Design review of the part built by this model. Coordinates are the model's own, in mm. A direction names the side the tool comes from. Coordinates: 2 decimals unless noted, no trailing zeros. Write each loop counter-clockwise with the first axis right and the second up, starting at its lowest first coordinate (ties: lowest second). Pieces come first, ordered by that corner, then holes. Notation, with made-up numbers: (-12, -17) -> (17, -17) arc R28 cw to (17, 17) -> close; hole circle Ø4 at (62, 9). An arc over 180 degrees is marked (long way). Write item = value, one per line. Start each with the question number.
```python
from build123d import *

# Parameters (mm, degrees)
SKETCH039_R     = 16.25
PAD017_DEPTH    = 4
POCKET014_DEPTH = 3.4
POCKET015_DEPTH = 0.601
CHAMFER012_SIZE = 0.4


with BuildPart() as part:
    # Sketch039 → Pad017 (new body)
    with BuildSketch(Plane.XY):
        with BuildLine():
            Line((-15.8267662036, 20.9422055079), (-4.8824534392, 29.2132101696))
            ThreePointArc((-4.8824534392, 29.2132101696), (-3.1285346801, 31.3265452468), (-2.5, 34))
            Line((-2.5, 34), (-2.5, 63.75))
            ThreePointArc((2.5, 63.75), (0, 66.25), (-2.5, 63.75))
            Line((2.5, 63.75), (2.5, 34))
            ThreePointArc((2.5, 34), (3.1285346801, 31.3265452468), (4.8824534392, 29.2132101696))
            Line((4.8824534392, 29.2132101696), (15.8267662036, 20.9422055079))
            ThreePointArc((-15.8267662036, 20.9422055079), (0, -26.25), (15.8267662036, 20.9422055079))
        make_face()
        Circle(SKETCH039_R, mode=Mode.SUBTRACT)
    extrude(amount=PAD017_DEPTH)

    # Sketch040 → Pocket014 (cut)
    with BuildSketch(Plane.XY):
        with BuildLine():
            Line((-14.9659183372, 6.3311759039), (-21.4611088655, 10.0811759039))
            ThreePointArc((-19.4611088655, 13.545277519), (-20.5342878135, 11.8554765967), (-21.4611088655, 10.0811759039))
            Line((-19.4611088655, 13.545277519), (-12.9659183372, 9.795277519))
            Line((-12.9659183372, 9.795277519), (-14.9659183372, 6.3311759039))
        make_face()
        with BuildLine():
            Line((-16.2287527148, 0.8307137431), (-23.6148108624, 2.1330750756))
            ThreePointArc((-22.9202181517, 6.0723060876), (-23.3507305362, 4.1173638128), (-23.6148108624, 2.1330750756))
            Line((-22.9202181517, 6.0723060876), (-15.5341600041, 4.7699447551))
            Line((-15.5341600041, 4.7699447551), (-16.2287527148, 0.8307137431))
        make_face()
        with BuildLine():
            Line((-11.8979733346, 11.0680048124), (-16.7188804073, 16.8133381358))
            ThreePointArc((-13.6547026348, 19.3844885746), (-15.2411069266, 18.1636439349), (-16.7188804073, 16.8133381358))
            Line((-13.6547026348, 19.3844885746), (-8.8337955622, 13.6391552512))
            Line((-11.8979733346, 11.0680048124), (-8.8337955622, 13.6391552512))
        make_face()
        with BuildLine():
            Line((-7.3949571526, 14.4698689943), (-9.9601082275, 21.5175636502))
            ThreePointArc((-6.2013377444, 22.8856442235), (-8.1096236096, 22.2810077477), (-9.9601082275, 21.5175636502))
            Line((-6.2013377444, 22.8856442235), (-3.6361866695, 15.8379495676))
            Line((-7.3949571526, 14.4698689943), (-3.6361866695, 15.8379495676))
        make_face()
        with BuildLine():
            Line((-15.5341600041, -4.7699447551), (-22.9202181517, -6.0723060876))
            ThreePointArc((-23.6148108624, -2.1330750756), (-23.3507305362, -4.1173638128), (-22.9202181517, -6.0723060876))
            Line((-23.6148108624, -2.1330750756), (-16.2287527148, -0.8307137431))
            Line((-16.2287527148, -0.8307137431), (-15.5341600041, -4.7699447551))
        make_face()
    extrude(amount=POCKET014_DEPTH, mode=Mode.SUBTRACT)

    # Pocket014 Face30 → Pocket015 (cut, through all)
    with BuildSketch(Plane(origin=(-19.6427739907, 3.4635510305, 3.4), x_dir=(0, -1, 0), z_dir=(0, 0, -1))):
        with BuildLine():
            Line((2.6328372874, -3.4140212759), (1.3304759549, 3.9720368717))
            ThreePointArc((1.3304759549, 3.9720368717), (-0.6538127823, 3.7079565456), (-2.6087550571, 3.277444161))
            Line((-2.6087550571, 3.277444161), (-1.3063937246, -4.1086139866))
            ThreePointArc((-1.3063937246, -4.1086139866), (0.6417681434, -3.6396480042), (2.6328372874, -3.4140212759))
        make_face()
    extrude(amount=-POCKET015_DEPTH, mode=Mode.SUBTRACT)

    # Chamfer012
    chamfer012_edges = [part.edges().sort_by_distance(p)[0] for p in [
        (2.41168, 16.070044, 4),
        (0, -26.25, 4),
        (0, -26.25, 0),
        (2.41168, -16.070044, 0),
        (-16.25, 0, 0),
        (-15.270005, 5.557827, 0),
        (-12.448222, 10.445299, 0),
        (-8.125, 14.072913, 0),
    ]]
    chamfer(chamfer012_edges, length=CHAMFER012_SIZE)


solid = part.part
```
(1) Mouldability with a two-part tool opening along Y and no side actions: class faces 1 (the face through (3.11, 31.36, 1.98)), 2 (the face through (-11.278, 16.552, 1.676)), 3 (the face through (2.5, 49, 2)) as pulls with the +Y half, pulls with the -Y half, needs draft (parallel to the pull), parting line crosses it, or undercut.
(2) Take a section at C-C, the plane z = 1.8. State the section outline as (x, y) points.
(3) Take a section at B-B, the plane x = 0. State the section outline as (y, z) points.
(4) For pin 1 Ø2 at (x, z) = (15.5, 2) entering from -Y; pin 2 Ø1.6 at (x, y) = (-21, -3) entering from -Z; pin 3 Ø12 at (x, y) = (-9, 44.5) entering from +Z, all flat-tipped, find the tip position at first contact; note any pin that passes through.
(5) Take a section at A-A, the plane y = 54. State the section outline as (x, z) points.
(6) For line 1 (Y direction, x = 0, z = 1.65); line 2 (X direction, y = 0, z = 1.85); line 3 (Y direction, x = -22.5, z = 0.3), list the stretches that pass through material, from the lowest coordinate up.
(7) For faces 4 (the face through (-18.2, 8.2, 1.7)), 5 (the face through (3.05, 31.24, 0.29)), 6 (the face through (-19.87, 1.473, 1.972)), list the 3-axis set-ups (+Z, -Z, +X, -X, +Y, -Y) from which the entire face can be reached by the end or side of a thin tool; tool diameter is ignored.
Report:
q1.face_1 = pulls with the +Y half
q1.face_2 = undercut
q1.face_3 = needs draft
q2.outline = (-15.83, 20.94) arc R26.25 ccw (long way) to (15.83, 20.94) -> (4.88, 29.21) arc R6 cw to (2.5, 34) -> (2.5, 63.75) arc R2.5 ccw to (-2.5, 63.75) -> (-2.5, 34) arc R6 cw to (-4.88, 29.21) -> close; hole (-23.61, -2.13) arc R23.71 ccw to (-22.92, -6.07) -> (-15.53, -4.77) arc R16.25 ccw (long way) to (-3.64, 15.84) -> (-6.2, 22.89) arc R23.71 ccw to (-9.96, 21.52) -> (-7.39, 14.47) arc R16.25 ccw to (-8.83, 13.64) -> (-13.65, 19.38) arc R23.71 ccw to (-16.72, 16.81) -> (-11.9, 11.07) arc R16.25 ccw to (-12.97, 9.8) -> (-19.46, 13.55) arc R23.71 ccw to (-21.46, 10.08) -> (-14.97, 6.33) arc R16.25 ccw to (-15.53, 4.77) -> (-22.92, 6.07) arc R23.71 ccw to (-23.61, 2.13) -> (-16.23, 0.83) arc R16.25 ccw to (-16.23, -0.83) -> close
q3.outline = (-26.25, 0.4) -> (-25.85, 0) -> (-16.65, 0) -> (-16.25, 0.4) -> (-16.25, 3.6) -> (-16.65, 4) -> (-25.85, 4) -> (-26.25, 3.6) -> close; (16.25, 0.4) -> (16.65, 0) -> (65.85, 0) -> (66.25, 0.4) -> (66.25, 3.6) -> (65.85, 4) -> (16.65, 4) -> (16.25, 3.6) -> close
q4.pin_1 = -21.88
q4.pin_2 = 3.4
q4.pin_3 = through
q5.outline = (-2.5, 0.4) -> (-2.1, 0) -> (2.1, 0) -> (2.5, 0.4) -> (2.5, 3.6) -> (2.1, 4) -> (-2.1, 4) -> (-2.5, 3.6) -> close
q6.line_1 = -26.25 to -16.25, 16.25 to 66.25
q6.line_2 = -26.25 to -16.25, 16.25 to 26.25
q6.line_3 = -13.33 to -6, -1.94 to 1.94, 6 to 13.33
q7.face_4 = -Z
q7.face_5 = -Z, +X, +Y
q7.face_6 = +Z, -Z
